```python
from build123d import *

# Parameters (mm, degrees)
SKETCH1_W           = 46.5
SKETCH1_H           = 23
BOSS_EXTRUDE1_DEPTH = 5
SKETCH2_W           = 44.5
SKETCH2_H           = 21
CUT_EXTRUDE1_DEPTH  = 4
SKETCH3_W           = 8
SKETCH3_H           = 5
BOSS_EXTRUDE2_DEPTH = 2.25
SKETCH4_R           = 1.625
CUT_EXTRUDE2_DEPTH  = 4.25
CHAMFER1_SIZE       = 1


with BuildPart() as part:
    # Sketch1 → Boss-Extrude1 (new body)
    with BuildSketch(Plane(origin=(0, 0, 0), x_dir=(1, 0, 0), z_dir=(0, 1, 0))):
        Rectangle(SKETCH1_W, SKETCH1_H)
    extrude(amount=BOSS_EXTRUDE1_DEPTH)

    # Sketch2 → Cut-Extrude1 (cut)
    with BuildSketch(Plane(origin=(0, 5, 0), x_dir=(1, 0, 0), z_dir=(0, 1, 0))):
        Rectangle(SKETCH2_W, SKETCH2_H)
    extrude(amount=-CUT_EXTRUDE1_DEPTH, mode=Mode.SUBTRACT)

    # Sketch3 → Boss-Extrude2 (add)
    with BuildSketch(Plane(origin=(0, 1, 0), x_dir=(1, 0, 0), z_dir=(0, 1, 0))):
        with Locations((-18.25, 8)):
            Rectangle(SKETCH3_W, SKETCH3_H)
        with Locations((18.25, 8)):
            Rectangle(SKETCH3_W, SKETCH3_H)
        with Locations((18.25, -8)):
            Rectangle(SKETCH3_W, SKETCH3_H)
        with Locations((-18.25, -8)):
            Rectangle(SKETCH3_W, SKETCH3_H)
    extrude(amount=BOSS_EXTRUDE2_DEPTH)

    # Sketch4 → Cut-Extrude2 (cut, through all)
    with BuildSketch(Plane(origin=(0, 3.25, 0), x_dir=(1, 0, 0), z_dir=(0, 1, 0))):
        with Locations((-16.5, 7.75)):
            Circle(SKETCH4_R)
        with Locations((16.5, 7.75)):
            Circle(SKETCH4_R)
        with Locations((16.5, -7.75)):
            Circle(SKETCH4_R)
        with Locations((-16.5, -7.75)):
            Circle(SKETCH4_R)
    extrude(amount=-CUT_EXTRUDE2_DEPTH, mode=Mode.SUBTRACT)

    # Chamfer1
    chamfer1_edges = [part.edges().sort_by_distance(p)[0] for p in [
        (0, 0, 11.5),
        (-23.25, 0, 0),
        (0, 0, -11.5),
        (23.25, 0, 0),
        (23.25, 2.5, 11.5),
        (-23.25, 2.5, 11.5),
        (-23.25, 2.5, -11.5),
        (23.25, 2.5, -11.5),
    ]]
    chamfer(chamfer1_edges, length=CHAMFER1_SIZE)


solid = part.part
```
Work out the finished part from the listing and answer in its coordinate system (mm). A direction names the side the tool comes from. Coordinates: 2 decimals unless noted, no trailing zeros. Loops run counter-clockwise (first coordinate to the right, second up) from the corner with the lowest first, then second, coordinate; pieces in that order, holes last. Notation, with made-up numbers: M -23.75,38 L 7.25,38 A22 cw 7.25,69 Z; hole C 70.25,27 d4. An arc over 180 degrees is marked long. Use CSV: the item, a comma, the result in double quotes. Start each with the question number.
(1) For faces 1 (the face through (23.25, 3, 0)), 2 (the face through (-18, 2, -5.5)), determine the directions among +Z, -Z, +X, -X, +Y, -Y from which every point of the face is accessible in a straight line to the end or side of a thin tool.
(2) Consider line 1 (Z direction, x = 16.5, y = 1.75) (3 decimals); line 2 (X direction, y = 2.35, z = 7.75) (3 decimals); line 3 (Z direction, x = 11.5, y = 2.75). Determine where each line is inside the solid, lowest interval first.
(3) Find section B-B, the plane z = -7.75. Give the vertices of the cut face in (x, y) (3 decimals).
(4) For a pull along X with two mould halves and no side action, classify faces 3 (the face through (-22.74, 2.97, 11.01)), 4 (the face through (18, 2, 5.5)), 5 (the face through (-14.25, 2, 8)), 6 (the face through (-2, 5, 11)) as +X half, -X half, draft (parallel to the pull), parting line (faces both ways), or undercut.
(5) Find section C-C, the plane y = 2.3. Give the vertices of the cut face in (x, z) (3 decimals), then the cut area to 3 significant figures.
(6) Find section A-A, the plane x = 16.5. Give the vertices of the cut face in (y, z) (3 decimals).
(7) Given pin 1 Ø2.5 at (x, z) = (-17, -7.5) entering from +Y; pin 2 Ø3 at (x, z) = (16.5, -7.75) entering from -Y; pin 3 Ø10 at (x, z) = (2, -3.5) entering from +Y, each flat-ended and moving along its own axis, determine where each tip first touches the part or whether it passes through.
(8) Find section D-D, the plane x = 11.5. Give the vertices of the cut face in (y, z).
Recorded:
1,face 1,"+Z, -Z, +X, +Y, -Y"
1,face 2,"+Y"
2,line 1,"z = -11.5 to -9.375, -6.125 to -5.5, 5.5 to 6.125, 9.375 to 11.5"
2,line 2,"x = -23.25 to -18.125, -14.875 to -14.25, 14.25 to 14.875, 18.125 to 23.25"
2,line 3,"z = -11.5 to -10.5, 10.5 to 11.5"
3,outline,"M -23.25,1 L -22.25,0 L -18.125,0 L -18.125,3.25 L -22.25,3.25 L -22.25,5 L -23.25,5 Z; M -14.875,0 L 14.875,0 L 14.875,3.25 L 14.25,3.25 L 14.25,1 L -14.25,1 L -14.25,3.25 L -14.875,3.25 Z; M 18.125,0 L 22.25,0 L 23.25,1 L 23.25,5 L 22.25,5 L 22.25,3.25 L 18.125,3.25 Z"
4,face 3,"-X half"
4,face 4,"undercut"
4,face 5,"undercut"
4,face 6,"draft"
5,outline,"M -23.25,-10.5 L -22.25,-11.5 L 22.25,-11.5 L 23.25,-10.5 L 23.25,10.5 L 22.25,11.5 L -22.25,11.5 L -23.25,10.5 Z; hole M -22.25,-5.5 L -14.25,-5.5 L -14.25,-10.5 L 14.25,-10.5 L 14.25,-5.5 L 22.25,-5.5 L 22.25,5.5 L 14.25,5.5 L 14.25,10.5 L -14.25,10.5 L -14.25,5.5 L -22.25,5.5 Z; hole C -16.5,-7.75 d3.25; hole C -16.5,7.75 d3.25; hole C 16.5,-7.75 d3.25; hole C 16.5,7.75 d3.25"
5,area,"260 mm^2"
6,outline,"M 0,-10.5 L 1,-11.5 L 5,-11.5 L 5,-10.5 L 3.25,-10.5 L 3.25,-9.375 L 0,-9.375 Z; M 0,-6.125 L 3.25,-6.125 L 3.25,-5.5 L 1,-5.5 L 1,5.5 L 3.25,5.5 L 3.25,6.125 L 0,6.125 Z; M 0,9.375 L 3.25,9.375 L 3.25,10.5 L 5,10.5 L 5,11.5 L 1,11.5 L 0,10.5 Z"
7,pin 1,"stops at y = 3.25"
7,pin 2,"passes through"
7,pin 3,"stops at y = 1"
8,outline,"M 0,-10.5 L 1,-11.5 L 5,-11.5 L 5,-10.5 L 1,-10.5 L 1,10.5 L 5,10.5 L 5,11.5 L 1,11.5 L 0,10.5 Z"
